```python
from build123d import *

# Parameters (mm, degrees)
SKETCH1_R                      = 17.5
BOSS_EXTRUDE1_DEPTH            = 4
SKETCH2_R                      = 12
BOSS_EXTRUDE2_DEPTH            = 0.6
CBORE_FOR_M3_SHCS1_D           = 3.2
CBORE_FOR_M3_SHCS1_CBORE_D     = 6.5
CBORE_FOR_M3_SHCS1_CBORE_DEPTH = 3
CHAMFER1_SIZE                  = 1


with BuildPart() as part:
    # Sketch1 → Boss-Extrude1 (new body)
    with BuildSketch(Plane.XY):
        Circle(SKETCH1_R)
    extrude(amount=BOSS_EXTRUDE1_DEPTH)

    # Sketch2 → Boss-Extrude2 (add)
    with BuildSketch(Plane(origin=(0, 0, 0), x_dir=(-1, 0, 0), z_dir=(0, 0, -1))):
        Circle(SKETCH2_R)
    extrude(amount=BOSS_EXTRUDE2_DEPTH)

    # CBORE for M3 SHCS1 (through all)
    with Locations(Plane.XY.offset(4)):
        with Locations((0, 8), (8, 0), (0, -8), (-8, 0)):
            CounterBoreHole(CBORE_FOR_M3_SHCS1_D / 2, CBORE_FOR_M3_SHCS1_CBORE_D / 2, CBORE_FOR_M3_SHCS1_CBORE_DEPTH)

    # Chamfer1
    chamfer1_edges = [part.edges().sort_by_distance(p)[0] for p in [
        (-17.5, 0, 4),
    ]]
    chamfer(chamfer1_edges, length=CHAMFER1_SIZE)


solid = part.part
```
The model under review builds one solid part; all positions refer to its coordinate system, in mm. A direction names the side the tool comes from. Coordinates: 2 decimals unless noted, no trailing zeros. Write each loop counter-clockwise with the first axis right and the second up, starting at its lowest first coordinate (ties: lowest second). Pieces come first, ordered by that corner, then holes.
1) We need section A-A on x = 0. State the section outline as (y, z) points, then the cut area to 3 significant figures.
2) Machinability: for faces 4 (the face through (0.35, 6.44, 0.19)), 5 (the face through (11.99, 0.53, -0.3)), 6 (the face through (9.4, -1.4, 1)), which of the approach directions +Z, -Z, +X, -X, +Y, -Y give a long, thin tool a straight path to every point of the face, cutting with its end or side? Answer none if there is none.
3) The part is to be moulded in two halves that separate along X. For faces 1 (the face through (-6.4, 0.07, 0.19)), 2 (the face through (0, 0, -0.6)), 3 (the face through (-13.887, -10.648, 1.479)), say which applies: pulls with the +X half, pulls with the -X half, needs draft (parallel to the pull), parting line crosses it, or undercut.
4) We need section C-C on z = 1.45. State the section outline as (x, y) points, then the cut area to 3 significant figures.
5) Clearance check with flat-ended pins moving along their axes: pin 1 Ø10.5 at (x, y) = (0, 8) entering from +Z; pin 2 Ø6 at (x, y) = (8, 0) entering from +Z; pin 3 Ø2.5 at (x, y) = (0, -8) entering from +Z; pin 4 Ø10 at (x, y) = (13.5, -13.5) entering from -Z. State where each tip first meets the part, or that it passes through.
6) To check wall thickness, follow probe 1 along Y at (x, z) = (0, -0.2); probe 2 along Y at (x, z) = (0, 2.15); probe 3 along Z at (x, y) = (6, 1). State the ranges of each line that lie inside material, in increasing order.
Answer list:
1. outline: (-17.5, 0) - (-12, 0) - (-12, -0.6) - (-9.6, -0.6) - (-9.6, 1) - (-11.25, 1) - (-11.25, 4) - (-16.5, 4) - (-17.5, 3) - close; (-6.4, -0.6) - (6.4, -0.6) - (6.4, 1) - (4.75, 1) - (4.75, 4) - (-4.75, 4) - (-4.75, 1) - (-6.4, 1) - close; (9.6, -0.6) - (12, -0.6) - (12, 0) - (17.5, 0) - (17.5, 3) - (16.5, 4) - (11.25, 4) - (11.25, 1) - (9.6, 1) - close
1. area: 104 mm2
2. face 4: +Z, -Z
2. face 5: -Z
2. face 6: +Z
3. face 1: undercut
3. face 2: needs draft
3. face 3: parting line crosses it
4. outline: circle Ø35 at (0, 0); hole circle Ø6.5 at (-8, 0); hole circle Ø6.5 at (0, -8); hole circle Ø6.5 at (0, 8); hole circle Ø6.5 at (8, 0)
4. area: 829 mm2
5. pin 1: stops at z = 4
5. pin 2: stops at z = 1
5. pin 3: passes through
5. pin 4: stops at z = 0
6. probe 1: y = -12 to -9.6, -6.4 to 6.4, 9.6 to 12
6. probe 2: y = -17.5 to -11.25, -4.75 to 4.75, 11.25 to 17.5
6. probe 3: z = -0.6 to 1
